Source: CAD feature listing. Evaluate the final solid. Frame: model axes, mm. Face numbers are marked on the shaded views. A direction names the side the tool comes from. Coordinates: 2 decimals unless noted, no trailing zeros. Write each loop counter-clockwise with the first axis right and the second up, starting at its lowest first coordinate (ties: lowest second). Pieces come first, ordered by that corner, then holes. Notation, with made-up numbers: M 48.5,11.5 L 53.5,11.5 A29 ccw 53.5,49.5 Z; hole C -3.5,35.25 d8. An arc over 180 degrees is marked long. Write item = value, one per line. Start each with the question number.
1. Line query: line 1 along Z through (x, y) = (-128, 69); line 2 along X through (y, z) = (89.5, 8.5); line 3 along X through (y, z) = (83, 54). Output: solid intervals per line, ascending.
2. Section query B-B (x = -166). Output: boundary loops of the cut face in (y, z), then the cut area to 3 significant figures.
3. Pull-direction query (Z, two-part tool) for the marked faces 1, 2 and 3; classes: pulls with the +Z half, pulls with the -Z half, needs draft (parallel to the pull), parting line crosses it, or undercut.
4. Section query A-A (y = 57). Output: boundary loops of the cut face in (x, z), then the cut area to 4 significant figures.
5. Access query for the marked faces 4, 5, 6, 7 and 8. Directions: +Z, -Z, +X, -X, +Y, -Y. A direction counts if a zero-diameter tool reaches every point of the face in a straight line with its end or side. Return the directions, or none.
6. Section query C-C (z = 40.5). Output: boundary loops of the cut face in (x, y).
7. Section query D-D (x = -116.5). Output: boundary loops of the cut face in (y, z).
8. Pin query (flat end, axial travel): pin 1 Ø5 at (x, z) = (-146, 7) entering from -Y; pin 2 Ø4 at (y, z) = (89.5, 66) entering from -X; pin 3 Ø4 at (x, z) = (-144.5, 53) entering from +Y. Return the tip coordinate at first contact, or that it passes through.
Autodesk Inventor part; units mm, degrees
ref_plane "Work Plane2" through (-162, -84, 44) normal (0, 0, 1) x (1, 0, 0)
ref_plane "YZ Plane" through (0, 0, 0) normal (1, 0, 0) x (0, 1, 0)
ref_plane "XZ Plane" through (0, 0, 0) normal (0, 1, 0) x (-1, 0, 0)
ref_plane "Work Plane1" through (0, 0, 0) normal (0, 0, 1) x (1, 0, 0)
ref_plane "Work Plane2" through (-162, -84, 44) normal (0, 0, 1) x (1, 0, 0)
sketch "Sketch1" plane through (0, 0, 0) normal (0, 0, 1) x (1, 0, 0)
  line L0 (-280, 0) -> (-160, 0)
  line L1 (-280, 0) -> (-280, -40)
  line L2 (-162, -40) -> (-280, -40)
  line L3 (-118, -40) -> (-162, -40)
  line L4 (0, -40) -> (-118, -40)
  line L5 (0, 0) -> (0, -40)
  line L6 (-120, 0) -> (0, 0)
  line L7 (-120, 0) -> (-120, 160)
  line L8 (0, 160) -> (-120, 160)
  line L9 (0, 160) -> (0, 200)
  line L10 (-280, 200) -> (0, 200)
  line L11 (-280, 160) -> (-280, 200)
  line L12 (-160, 160) -> (-280, 160)
  line L13 (-160, 0) -> (-160, 160)
  line L14 (-160, 87.5) -> (-120, 87.5)
  line L15 (-120, 87.5) -> (-120, 72.5)
  line L16 (-120, 72.5) -> (-160, 72.5)
  line L17 (-160, 72.5) -> (-160, 87.5)
  line L18 (-160, 87.5) -> (-120, 72.5) construction
  line L19 (-120, 87.5) -> (-160, 72.5) construction
  point P0 (-140, 80)
  dimension "d0" = 40
  dimension "d1" = 15
extrude "Extrusion1" add sketch "Sketch1" along normal up to surface (44 mm away) contours L13 L14 L7 L16
ref_plane "Work Plane3" through (0, 0, 0) normal (0, 0, 1) x (1, 0, 0)
sketch "Sketch2" plane through (0, 0, 0) normal (0, 0, 1) x (1, 0, 0)
  line L0 (-120, 87.5) -> (-120, 72.5)
  line L1 (-160, 87.5) -> (-120, 87.5)
  line L2 (-160, 72.5) -> (-160, 87.5)
  line L3 (-120, 72.5) -> (-160, 72.5)
  line L4 (-160, 105) -> (-120, 105)
  line L5 (-120, 105) -> (-120, 55)
  line L6 (-120, 55) -> (-160, 55)
  line L7 (-160, 55) -> (-160, 105)
  line L8 (-160, 105) -> (-120, 55) construction
  line L9 (-120, 105) -> (-160, 55) construction
  point P0 (0, 0)
  point P1 (-140, 80)
  dimension "d7" = 40
  dimension "d8" = 50
extrude "Extrusion2" add sketch "Sketch2" along normal blind 10 contours L1 L7 L4 L5 | L5 L6 L7 L3
sketch "Sketch3" plane through (-160, 87.5, 44) normal (0, 1, 0) x (1, 0, 0)
  line L0 (0, 0) -> (55, 0)
  line L1 (55, 0) -> (55, -21)
  line L2 (55, -21) -> (0, -21)
  line L3 (0, -21) -> (0, 0)
  point P0 (160, 44)
  dimension "d11" = 55
  dimension "d12" = 21
extrude "Extrusion3" add sketch "Sketch3" against normal blind 40
sketch "Sketch4" plane through (-160, 87.5, 10) normal (0, 1, 0) x (1, 0, 0)
  line L0 (40, 0) -> (0, 0)
  line L1 (0, 0) -> (0, -55)
  line L2 (55, -55) -> (0, -55)
  line L3 (55, -34) -> (55, -55)
  line L4 (40, -34) -> (55, -34)
  line L5 (40, 0) -> (40, -34)
  line L6 (55, -55) -> (0, -55)
  line L7 (55, -34) -> (0, -34)
  line L8 (0, -34) -> (0, -55)
  line L9 (0, -55) -> (55, -55)
  line L10 (55, -55) -> (55, -34)
  line L11 (0, -44.5) -> (15, -44.5)
  line L12 (0, -44.5) -> (15, -44.5) construction
  circle A0 centre (15, -44.5) radius 4
  point P0 (160, 10)
  dimension "d15" = 15
  dimension "d16" = 0
  dimension "d17" = 8
extrude "Extrusion4" add sketch "Sketch4" along normal blind 8 contours A0
sketch "Sketch5" plane through (-160, 87.5, 10) normal (0, 1, 0) x (1, 0, 0)
  circle A0 centre (15, -44.5) radius 4
  line L0 (40, 0) -> (0, 0)
  line L1 (0, 0) -> (0, -55)
  line L2 (55, -55) -> (0, -55)
  line L3 (55, -34) -> (55, -55)
  line L4 (40, -34) -> (55, -34)
  line L5 (40, 0) -> (40, -34)
  circle A1 centre (15, -44.5) radius 4
  line L6 (15, -44.5) -> (28, -44.5)
  line L7 (15, -44.5) -> (28, -44.5) construction
  line L8 (15, -44.5) -> (2, -44.5)
  line L9 (15, -44.5) -> (28, -44.5) construction
  line L10 (28, -44.5) -> (38, -44.5)
  line L11 (38, -44.5) -> (38, -84.5)
  line L12 (38, -84.5) -> (28, -84.5)
  line L13 (28, -84.5) -> (28, -44.5)
  line L14 (28, -44.5) -> (23, -44.5)
  line L15 (23, -44.5) -> (23, -84.5)
  line L16 (23, -84.5) -> (28, -84.5)
  line L17 (28, -84.5) -> (28, -44.5)
  line L18 (3.5452, -38.0217) -> (16.5356, -45.5217)
  line L19 (16.5356, -45.5217) -> (-3.4644, -80.1628)
  line L20 (-3.4644, -80.1628) -> (-16.4548, -72.6628)
  line L21 (-16.4548, -72.6628) -> (3.5452, -38.0217)
  line L22 (3.5452, -38.0217) -> (8.5452, -29.3615)
  line L23 (8.5452, -29.3615) -> (21.5356, -36.8615)
  line L24 (21.5356, -36.8615) -> (16.5356, -45.5217)
  point P0 (160, 10)
  dimension "d20" = 13
  dimension "d21" = 0
  dimension "d22" = 13
  dimension "d23" = 180
  dimension "d24" = 10
  dimension "d25" = 40
  dimension "d26" = 5
  dimension "d27" = 15
  dimension "d28" = 40
  dimension "d31" = 10
extrude "Extrusion5" add sketch "Sketch5" along normal blind 5 contours L24 L6 L8 L18 A0 | A0 L18 L22 L23 L24 | L19 L2 L1 L21 L18 A0 | A0 L8 L18 L19 | L6 L13 L2 L15 | L24 L18 L8 L6 | L18 L8 A0 | L19 L20 L21 L1 L2 | L10 L11 L2 L13 | L2 L13 L16 L15 | L2 L11 L12 L13
sketch "Sketch6" plane through (-160, 92.5, 10) normal (0, 1, 0) x (1, 0, 0)
  line L0 (23, -84.5) -> (38, -84.5)
  line L1 (38, -84.5) -> (38, -44.5)
  line L2 (38, -44.5) -> (23, -44.5)
  line L3 (23, -44.5) -> (23, -84.5)
  arc A0 (18.3698, -42.3448) -> (14.8185, -48.4959) centre (15, -44.5) ccw
  line L4 (18.3698, -42.3448) -> (21.5356, -36.8615)
  line L5 (21.5356, -36.8615) -> (8.5452, -29.3615)
  line L6 (8.5452, -29.3615) -> (-16.4548, -72.6628)
  line L7 (-16.4548, -72.6628) -> (-3.4644, -80.1628)
  line L8 (-3.4644, -80.1628) -> (14.8185, -48.4959)
  circle A1 centre (15, -44.5) radius 4
  line L9 (15, -44.5) -> (15, -71.5)
  circle A2 centre (15, -71.5) radius 13
  line L10 (15, -44.5) -> (3.1255, -68.7486)
  circle A3 centre (3.1255, -68.7486) radius 13
  point P0 (160, 10)
  dimension "d32" = 27
  dimension "d33" = 26
  dimension "d34" = 27
  dimension "d35" = 26
extrude "Extrusion6" cut sketch "Sketch6" against normal blind 5 contours A2 A3 L9 L3 | L3 A2 | A3 L8 A2 | A2 L8 A3 | L9 A3 A2 | A2 L10 L8 | L8 A3 L10 A2 | A2 L8 A3 | L10 A2 L8 | L10 A3 L8 A2
equation "\"d34\" = d32"
equation "\"d35\" = d33"
properties part number "BSF_ShuttleFeeder"
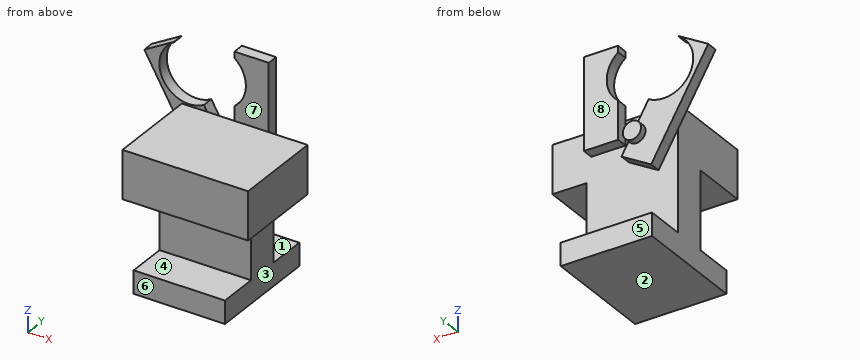
Results are:
q1.line_1 = 0 to 10, 44 to 65
q1.line_2 = -160 to -120
q1.line_3 = -160 to -105
q2.outline = M 87.5,64.55 L 92.5,64.55 L 92.5,69.49 L 87.5,69.49 Z; M 87.5,88.01 L 92.5,88.01 L 92.5,88.7 L 87.5,88.7 Z
q2.area = 28.1 mm^2
q3.face_1 = undercut
q3.face_2 = pulls with the -Z half
q3.face_3 = needs draft
q4.outline = M -160,0 L -120,0 L -120,10 L -160,10 Z; M -160,44 L -105,44 L -105,65 L -160,65 Z
q4.area = 1,555 mm^2
q5.face_4 = +X, -X, -Y
q5.face_5 = +Z, -Z, +X, -X, +Y
q5.face_6 = -Z, +X, -X, -Y
q5.face_7 = +Z, +X, -X, -Y
q5.face_8 = +Z, +X, +Y
q6.outline = M -160,72.5 L -120,72.5 L -120,87.5 L -149.48,87.5 L -149.48,92.5 L -152.11,92.5 L -152.11,87.5 L -160,87.5 Z
q7.outline = M 47.5,44 L 87.5,44 L 87.5,65 L 47.5,65 Z
q8.pin_1 = 55
q8.pin_2 = -167.99
q8.pin_3 = 95.5
